Geometry: final body of the model. Coordinates: model frame, mm. A direction names the side the tool comes from. Give positions to 0.01 mm unless a question says otherwise; leave off trailing zeros. Loops run counter-clockwise (first coordinate to the right, second up) from the corner with the lowest first, then second, coordinate; pieces in that order, holes last.
```python
from build123d import *

# Parameters (mm, degrees)
F0_R     = 29
F1_DEPTH = 25
F2_R     = 10.5
F3_DEPTH = 10
F5_D     = 11.1
F9_D     = 2.5
F13_D    = 2.5


with BuildPart() as f1:
    # F0 (on Top) → F1 (new body)
    with BuildSketch(Plane.XY):
        Circle(F0_R)
    extrude(amount=F1_DEPTH)

    # F2 (on face) → F3 (join)
    with BuildSketch(Plane(origin=(0, 0, 0), x_dir=(1, 0, 0), z_dir=(0, 0, -1))):
        Circle(F2_R)
    extrude(amount=F3_DEPTH)

    # F5 (through all)
    with Locations(Plane(origin=(0, 0, -10), x_dir=(1, 0, 0), z_dir=(0, 0, -1))):
        with Locations((0, 0)):
            Hole(F5_D / 2)

    # F9 (through all)
    with Locations(Plane(origin=(-10.5, 0, 0), x_dir=(0, -1, 0), z_dir=(-1, 0, 0))):
        with Locations((0, -5.3152111359)):
            Hole(F9_D / 2)

    # F13 (through all)
    with Locations(Plane(origin=(0, 10.5, 0), x_dir=(-1, 0, 0), z_dir=(0, 1, 0))):
        with Locations((0, -4.9469849671)):
            Hole(F13_D / 2)


solid = f1.part
```
Q1. Section query D-D, the plane y = 9. Return loops of the section in (x, z), and give its area (3 significant figures).
Q2. Material intervals for probe 1 along Z at (x, y) = (8, 0); probe 2 along Z at (x, y) = (0, 6); probe 3 along Y at (x, z) = (0, 0.5), sorted ascending.
Q3. Reachability of faces 4 (the face through (12, 0, 0)), 5 (the face through (-0.271, 7.917, -6.167)) from +Z, -Z, +X, -X, +Y, -Y: full face, straight path, thin tool, end or side. Return the list, or none.
Q4. Section query A-A, the plane x = 0. Return loops of the section in (y, z).
Q5. Mould query, pull axis X, two halves, no side actions, for faces 1 (the face through (13.38, -25.73, 12.32)), 2 (the face through (-0.271, -7.989, -6.167)), 3 (the face through (6, 0, 25)). Classes: +X half, -X half, draft (parallel to the pull), parting line (faces both ways), or undercut.
Q6. Section query C-C, the plane z = 9.5. Return loops of the section in (x, y).
Q7. Section query B-B, the plane y = 0. Return loops of the section in (x, z), and give its area (3 significant figures).
Q8. Pin query (flat end, axial travel): pin 1 Ø4 at (x, z) = (-5, 16.5) entering from +Y; pin 2 Ø10 at (x, z) = (-0.5, 13) entering from -Y; pin 3 Ø8 at (y, z) = (11.5, 8.5) entering from -X; pin 4 Ø12 at (x, y) = (2.5, -0.5) entering from -Z. Return the tip coordinate at first contact, or that it passes through.
Resolved:
1. outline: (-27.57, 0) - (-5.41, 0) - (-5.41, -10) - (5.41, -10) - (5.41, 0) - (27.57, 0) - (27.57, 25) - (-27.57, 25) - close; hole circle Ø2.5 at (0, -4.95)
1. area: 1,480 mm2
2. probe 1: z = -10 to -6.57, -4.07 to 25
2. probe 2: z = -10 to -6.2, -3.7 to 25
2. probe 3: y = -29 to -5.55, 5.55 to 29
3. face 4: -Z
3. face 5: +Y, -Y
4. outline: (-29, 0) - (-10.5, 0) - (-10.5, -3.7) - (-5.55, -3.7) - (-5.55, 25) - (-29, 25) - close; (-10.5, -10) - (-5.55, -10) - (-5.55, -6.2) - (-10.5, -6.2) - close; (5.55, -10) - (10.5, -10) - (10.5, -6.2) - (5.55, -6.2) - close; (5.55, -3.7) - (10.5, -3.7) - (10.5, 0) - (29, 0) - (29, 25) - (5.55, 25) - close
5. face 1: parting line
5. face 2: undercut
5. face 3: draft
6. outline: circle Ø58 at (0, 0); hole circle Ø11.1 at (0, 0)
7. outline: (-29, 0) - (-10.5, 0) - (-10.5, -4.07) - (-5.55, -4.07) - (-5.55, 25) - (-29, 25) - close; (-10.5, -10) - (-5.55, -10) - (-5.55, -6.57) - (-10.5, -6.57) - close; (5.55, -10) - (10.5, -10) - (10.5, -6.57) - (5.55, -6.57) - close; (5.55, -4.07) - (10.5, -4.07) - (10.5, 0) - (29, 0) - (29, 25) - (5.55, 25) - close
7. area: 1,250 mm2
8. pin 1: stops at y = 28.84
8. pin 2: stops at y = -29
8. pin 3: stops at x = -28.01
8. pin 4: stops at z = -10
